Build history of the part. All positions in model axes, mm. A direction names the side the tool comes from. Coordinates: 2 decimals unless noted, no trailing zeros. Write each loop counter-clockwise with the first axis right and the second up, starting at its lowest first coordinate (ties: lowest second). Pieces come first, ordered by that corner, then holes.
Autodesk Inventor part; units mm, degrees
ref_plane "YZ Plane" through (0, 0, 0) normal (1, 0, 0) x (0, 1, 0)
ref_plane "XZ Plane" through (0, 0, 0) normal (0, 1, 0) x (-1, 0, 0)
ref_plane "XY Plane" through (0, 0, 0) normal (0, 0, 1) x (1, 0, 0)
sketch "Sketch1" plane through (0, 0, 0) normal (0, 1, 0) x (-1, 0, 0)
  circle A0 centre (0, 0) radius 30
  circle A1 centre (0, 0) radius 39 construction
  circle A2 centre (0, 0) radius 80
  circle A3 centre (39, 0) radius 5.1
  circle A4 centre (19.5, 33.775) radius 5.1
  circle A5 centre (-19.5, 33.775) radius 5.1
  circle A6 centre (-39, 0) radius 5.1
  circle A7 centre (-19.5, -33.775) radius 5.1
  circle A8 centre (19.5, -33.775) radius 5.1
  dimension "d0" = 78
  dimension "d1" = 160
  dimension "d2" = 60
  dimension "d3" = 10.2
  dimension "d6" = 360
extrude "Extrusion1" add sketch "Sketch1" along normal blind 20
sketch "Sketch2" plane through (0, 20, 0) normal (0, 1, 0) x (1, 0, 0)
  circle A0 centre (0, 0) radius 30 construction
  circle A1 centre (-19.5, 33.775) radius 5.1 construction
  circle A2 centre (19.5, 33.775) radius 5.1 construction
  circle A3 centre (39, 0) radius 5.1 construction
  circle A4 centre (19.5, -33.775) radius 5.1 construction
  circle A5 centre (-19.5, -33.775) radius 5.1 construction
  circle A6 centre (-39, 0) radius 5.1 construction
  circle A7 centre (0, 0) radius 80 construction
  line L0 (0, -80) -> (0, 80) construction
  line L1 (-18, 80) -> (18, 80)
  line L2 (18, 80) -> (18, 44)
  line L3 (18, 44) -> (-18, 44)
  line L4 (-18, 44) -> (-18, 80)
  circle A8 centre (0, 0) radius 80 construction
  circle A9 centre (0, 62) radius 5.05
  dimension "d10" = 36
  dimension "d11" = 10.1
  dimension "d12" = 18
  dimension "d13" = 36
extrude "Extrusion2" cut sketch "Sketch2" against normal blind 10
extrude "Extrusion3" cut sketch "Sketch2" against normal through all contours A9
pattern_circular "Circular Pattern1" count 6 over 360 about axis through (0, 0, 0) along (0, 1, 0) of "Extrusion2", "Extrusion3"
properties part number "terminal-cap"
(1) Slice it at C-C, the plane x = 37. List the corners of the cut face in (y, z).
(2) Slice it at A-A, the plane x = 1. List the corners of the cut face in (y, z), and give its area (3 significant figures).
(3) Flat gauge pins, fed straight in: P1, Ø6, axis at x = 19.5, z = -33.775, coming from the -Y side; P2, Ø3, axis at y = 14.5, z = 59.5, coming from the -X side; P3, Ø5, axis at y = 16, z = 66.5, coming from the +X side; P4, Ø8, axis at x = -59.5, y = 11.5, coming from the -Z side. Where does each tip first touch, or does it go through?
(4) Slice it at D-D, the plane y = 14. Give the number of separate pieces and of enclosed holes in the cut face, and give its area (3 significant figures).
(5) Two-plate mould, pull along Z, no slides. Class faces 1 (the flat face through (18, 15, 61)), 2 (the flat face through (-37.98, 15.07, -22.22)), 3 (the cylindrical face through (17.34, 7.64, 78.1)): pulls with the +Z half, pulls with the -Z half, needs draft (parallel to the pull), parting line crosses it, or undercut.
(6) 3-axis set-ups, long thin cutter, end or side, ignore diameter. For faces 4 (the flat face through (61.6, 15.07, 14.78)), 5 (the flat face through (-4, 10, 66)), 6 (the flat face through (-18, 15, -61)), 7 (the flat face through (44.011, 15.07, 46.194)): which of +Z, -Z, +X, -X, +Y, -Y reach the whole face in a straight line?
(7) Probe L1, parallel to Z at x = 51.5, y = 5.75; L2, parallel to Z at x = 19.5, y = 4.25 (3 decimals); L3, parallel to Z at x = -32.5, y = 18.5. List the from-to ranges inside material, lowest first.
(8) Slice it at B-B, the plane z = 62. List the corners of the cut face in (x, y), and give its area (3 significant figures).
Results:
1. outline: (0, -70.93) - (20, -70.93) - (20, -42.15) - (10, -42.15) - (10, -23.91) - (20, -23.91) - (20, -4.69) - (0, -4.69) - close; (0, 4.69) - (20, 4.69) - (20, 23.91) - (10, 23.91) - (10, 42.15) - (20, 42.15) - (20, 70.93) - (0, 70.93) - close
2. outline: (0, -79.99) - (10, -79.99) - (10, -66.95) - (0, -66.95) - close; (0, -57.05) - (10, -57.05) - (10, -44) - (20, -44) - (20, -29.98) - (0, -29.98) - close; (0, 29.98) - (20, 29.98) - (20, 44) - (10, 44) - (10, 57.05) - (0, 57.05) - close; (0, 66.95) - (10, 66.95) - (10, 79.99) - (0, 79.99) - close
2. area: 1,080 mm2
3. P1: passes through
3. P2: stops at x = -55.1
3. P3: stops at x = 48
3. P4: stops at z = -57.62
4. separate pieces: 1
4. enclosed holes: 7
4. area: 9,160 mm2
5. face 1: needs draft
5. face 2: undercut
5. face 3: parting line crosses it
6. face 4: +Y
6. face 5: +Z, +Y
6. face 6: -Z, +Y
6. face 7: +X, +Y
7. L1: z = -61.22 to -35.55, -26.45 to 26.45, 35.55 to 61.22
7. L2: z = -77.587 to -38.875, -28.675 to -22.798, 22.798 to 28.675, 38.875 to 77.587
7. L3: z = -73.1 to -39.55, -31.71 to 31.71, 39.55 to 73.1
8. outline: (-50.56, 0) - (-5.05, 0) - (-5.05, 10) - (-18, 10) - (-18, 20) - (-50.56, 20) - close; (5.05, 0) - (50.56, 0) - (50.56, 20) - (18, 20) - (18, 10) - (5.05, 10) - close
8. area: 1,560 mm2
